Verification items for the finished model (mm, model axes). Face numbers are marked on the shaded views. A direction names the side the tool comes from. Give positions to 0.01 mm unless a question says otherwise; leave off trailing zeros. Order: outer loops, then holes, each group sorted by start corner. A loop starts at its lowest first (then second) coordinate and runs counter-clockwise, first axis right, second up. Notation, with made-up numbers: (-27, 5.25) -> (25, 5.25) arc R18 cw to (25, 25.25) -> close; hole circle Ø5 at (-21, 36.5). An arc over 180 degrees is marked (long way). One line per question, with ' | ' between items. Start each with the question number.
Q1. Go/stop test with flat-tipped pins: pin 1 (12 mm diameter, centred on x = -29.5, y = 13.5, fed in from +Z); pin 2 (1.5 mm diameter, centred on x = -36, y = 8, fed in from +Z); pin 3 (3 mm diameter, centred on y = 0.5, z = 9, fed in from -X). Record where each tip stops, or that it passes through.
Q2. Section check B-B on x = -48. Record the cut outline in (y, z), plus the area to 4 significant figures.
Q3. Section check A-A on y = 26. Record the cut outline in (x, z).
Q4. Access from +Z, -Z, +X, -X, +Y, -Y to the whole of each face (thin tool, end or side, straight path). Record for the marked faces 1 and 2.
Q5. Section check D-D on y = 4.5. Record the cut outline in (x, z), plus the area to 3 significant figures.
Q6. Material ranges on probe 1 along X at (y, z) = (-11.5, 6.25); probe 2 along X at (y, z) = (10.5, 8); probe 3 along Y at (x, z) = (-48, 1.9), recorded low to high. Write a range as [from, to].
Q7. Section check C-C on z = 12.25. Record the cut outline in (x, y).
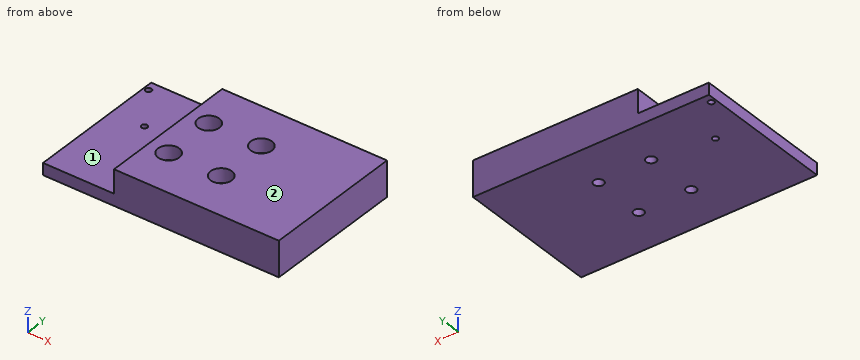
from build123d import *

# Parameters (mm, degrees)
SKETCH_1_W                = 100
SKETCH_1_H                = 60
EXTRUDE_1_DEPTH           = 15
HOLE_WIZARD_9_0_9_1_D     = 9
HOLE_WIZARD_9_0_9_1_DEPTH = 6
HOLE_WIZARD_9_0_9_1_TIP   = 2.703872786
HOLE_WIZARD_M5_2_D        = 4.2
SKETCH_8_W                = 30.11564459
SKETCH_8_H                = 60
CUT_EXTRUDE_2_DEPTH       = 10
HOLE_WIZARD_M3_1_D        = 2.5


with BuildPart() as part:
    # 스케치1 → 보스-돌출1 (new body)
    with BuildSketch(Plane.XY):
        Rectangle(SKETCH_1_W, SKETCH_1_H)
    extrude(amount=EXTRUDE_1_DEPTH)

    # Ø9.0 (9) 지름 구멍1
    with Locations(Plane(origin=(-11.136931804, 11.136931804, 15), x_dir=(1, 0, 0), z_dir=(0, 0, 1))):
        with Locations((0, 0), (22.273863608, 0), (0, -22.273863608), (22.273863608, -22.273863608)):
            Hole(HOLE_WIZARD_9_0_9_1_D / 2, depth=HOLE_WIZARD_9_0_9_1_DEPTH)
            with Locations((0, 0, -(HOLE_WIZARD_9_0_9_1_DEPTH + HOLE_WIZARD_9_0_9_1_TIP / 2))):  # 118° drill point
                Cone(0, HOLE_WIZARD_9_0_9_1_D / 2, HOLE_WIZARD_9_0_9_1_TIP, mode=Mode.SUBTRACT)

    # M5 나사 구멍2 (through all)
    with Locations(Plane.XY.offset(15)):
        with Locations((-11.136931804, 11.136931804), (11.136931804, 11.136931804), (11.136931804, -11.136931804), (-11.136931804, -11.136931804)):
            Hole(HOLE_WIZARD_M5_2_D / 2)

    # 스케치8 → 컷-돌출2 (cut)
    with BuildSketch(Plane.XY.offset(15)):
        with Locations((-34.942177705, 0)):
            Rectangle(SKETCH_8_W, SKETCH_8_H)
    extrude(amount=-CUT_EXTRUDE_2_DEPTH, mode=Mode.SUBTRACT)

    # M3 나사 구멍1 (through all)
    with Locations(Plane(origin=(-36, 8, 0), x_dir=(-1, 0, 0), z_dir=(0, 0, -1))):
        with Locations((0, 0), (12, 18)):
            Hole(HOLE_WIZARD_M3_1_D / 2)


solid = part.part
Filled in:
1) pin 1: z = 5 | pin 2: through | pin 3: x = -19.88
2) outline: (-30, 0) -> (24.75, 0) -> (24.75, 5) -> (-30, 5) -> close; (27.25, 0) -> (30, 0) -> (30, 5) -> (27.25, 5) -> close | area: 287.5 mm²
3) outline: (-50, 0) -> (-49.25, 0) -> (-49.25, 5) -> (-50, 5) -> close; (-46.75, 0) -> (50, 0) -> (50, 15) -> (-19.88, 15) -> (-19.88, 5) -> (-46.75, 5) -> close
4) face 1: +Z, -X, +Y, -Y | face 2: +Z, +X, -X, +Y, -Y
5) outline: (-50, 0) -> (50, 0) -> (50, 15) -> (-19.88, 15) -> (-19.88, 5) -> (-50, 5) -> close | area: 1,200 mm²
6) probe 1: [-19.88, -13.21], [-9.07, 9.07], [13.21, 50] | probe 2: [-19.88, -13.9], [-8.37, 8.37], [13.9, 50] | probe 3: [-30, 24.75], [27.25, 30]
7) outline: (-19.88, -30) -> (50, -30) -> (50, 30) -> (-19.88, 30) -> close; hole circle Ø9 at (-11.14, -11.14); hole circle Ø9 at (-11.14, 11.14); hole circle Ø9 at (11.14, -11.14); hole circle Ø9 at (11.14, 11.14)
